```python
from build123d import *
from build123d.topology import SkipClean

# Parameters (mm, degrees)
SKETCH1_R           = 3.2512
SKETCH1_R_2         = 1.4732
SKETCH1_R_3         = 2.2987
BOSS_EXTRUDE1_DEPTH = 3.81
CUT_EXTRUDE2_START  = -1.651
CUT_EXTRUDE2_DEPTH  = 1.651


with BuildPart() as part:
    # Sketch1 → Boss-Extrude1 (new body)
    with BuildSketch(Plane.XY):
        with BuildLine():
            Line((7.944916334, 12.956699963), (-7.685191608, 2.536045689))
            ThreePointArc((-7.685191608, 2.536045689), (-9.0424, 0), (-7.685191608, -2.536045689))
            Line((-7.685191608, -2.536045689), (7.944916334, -12.956699963))
            ThreePointArc((7.944916334, -12.956699963), (13.779763951, -12.157804059), (13.70040037, -6.26905353))
            ThreePointArc((13.70040037, -6.26905353), (11.2776, 0), (13.70040037, 6.26905353))
            ThreePointArc((13.70040037, 6.26905353), (13.779763951, 12.157804059), (7.944916334, 12.956699963))
        make_face()
        with Locations(Location((0, 0, 0), (0, 0, 180))):
            Circle(SKETCH1_R, mode=Mode.SUBTRACT)
        with Locations(Location((-5.9944, 0, 0), (0, 0, 180))):
            Circle(SKETCH1_R_2, mode=Mode.SUBTRACT)
        with Locations(Location((5.9944, 0, 0), (0, 0, 180))):
            Circle(SKETCH1_R_2, mode=Mode.SUBTRACT)
        with Locations(Location((10.410654097, 9.2583, 0), (0, 0, 180))):
            Circle(SKETCH1_R_3, mode=Mode.SUBTRACT)
        with Locations(Location((10.410654097, -9.2583, 0), (0, 0, 180))):
            Circle(SKETCH1_R_3, mode=Mode.SUBTRACT)
    extrude(amount=BOSS_EXTRUDE1_DEPTH)

    # Sketch2 → Cut-Extrude2 (cut)
    with SkipClean():  # the faces are left unmerged after this step: merging them gives an invalid solid
        with BuildSketch(Plane.XY.offset(3.81).offset(CUT_EXTRUDE2_START)):
            with BuildLine():
                Line((7.944916334, 12.956699963), (-7.685191608, 2.536045689))
                ThreePointArc((-7.685191608, 2.536045689), (-9.0424, 0), (-7.685191608, -2.536045689))
                Line((-7.685191608, -2.536045689), (7.944916334, -12.956699963))
                ThreePointArc((7.944916334, -12.956699963), (7.041544243, -6.358795941), (13.70040037, -6.26905353))
                ThreePointArc((13.70040037, -6.26905353), (11.2776, 0), (13.70040037, 6.26905353))
                ThreePointArc((13.70040037, 6.26905353), (7.041544243, 6.358795941), (7.944916334, 12.956699963))
            make_face()
        extrude(amount=CUT_EXTRUDE2_DEPTH, mode=Mode.SUBTRACT)


solid = part.part
```
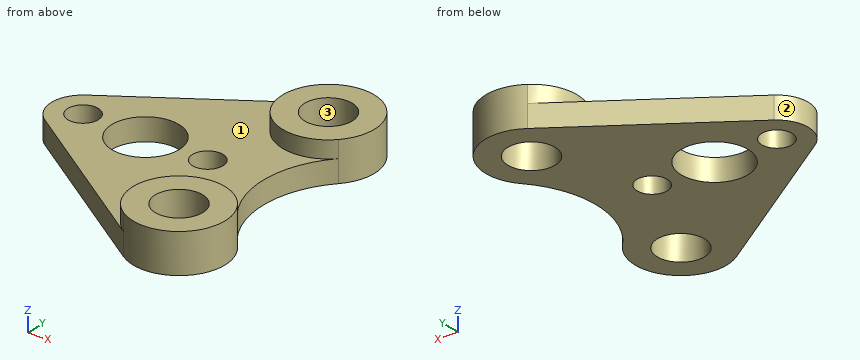
CAD build for the part. Positions are in the model's coordinates, mm. Face numbers are marked on the shaded views. Coordinates: 2 decimals unless noted, no trailing zeros. Write each loop counter-clockwise with the first axis right and the second up, starting at its lowest first coordinate (ties: lowest second). Pieces come first, ordered by that corner, then holes. Notation, with made-up numbers: (33.5, 26) -> (77.5, 26) arc R24 ccw to (77.5, 46) -> close; hole circle Ø9 at (26.5, 17.5). An arc over 180 degrees is marked (long way). Return JSON: item names as keys, results as strings. Group by question number.
Q1. Drill centre lines: line 1 (Y direction, x = 12.5, z = 2.75); line 2 (Y direction, x = 9.5, z = 2); line 3 (Y direction, x = 9.75, z = 2.5). Where is each one in solid material? Low to high.
Q2. Cut at B-B, the plane x = 10.75. Give the cut face in (y, z).
Q3. Cut at D-D, the plane x = 0. Give the cut face in (y, z).
Q4. Cut at C-C, the plane z = 3.1. Give the cut face in (x, y) (3 decimals), then the cut area to 3 significant figures.
Q5. Cut at A-A, the plane y = 0. Give the cut face in (x, z).
Q6. Flat gauge pins, fed straight in: pin 1 (1.5 mm diameter, centred on x = -3.5, z = 2.5, fed in from -Y); pin 2 (5 mm diameter, centred on x = 0, y = 0, fed in from +Z); pin 3 (1.5 mm diameter, centred on y = -1, z = 2, fed in from +X); pin 4 (7 mm diameter, centred on x = -3, y = 4.5, fed in from +Z). Where does each tip first touch, or does it go through?
Q7. Pull direction X, two halves, no side cores. Call the marked faces 1, 2 and 3: released by +X, released by -X, zero draft, split by the parting line, or undercut.
Returned:
{
 "1": {"line 1": "y = -13.18 to -10.22, -8.3 to -5.33, 5.33 to 8.3, 10.22 to 13.18", "line 2": "y = -13.61 to -11.37, -7.15 to 7.15, 11.37 to 13.61", "line 3": "y = -13.65 to -11.46, -7.06 to -4.86, 4.86 to 7.06, 11.46 to 13.65"},
 "2": {"outline": "(-13.69, 0) -> (-11.53, 0) -> (-11.53, 3.81) -> (-13.69, 3.81) -> close; (-6.98, 0) -> (6.98, 0) -> (6.98, 3.81) -> (4.83, 3.81) -> (4.83, 2.16) -> (-4.83, 2.16) -> (-4.83, 3.81) -> (-6.98, 3.81) -> close; (11.53, 0) -> (13.69, 0) -> (13.69, 3.81) -> (11.53, 3.81) -> close"},
 "3": {"outline": "(-7.66, 0) -> (-3.25, 0) -> (-3.25, 2.16) -> (-7.66, 2.16) -> close; (3.25, 0) -> (7.66, 0) -> (7.66, 2.16) -> (3.25, 2.16) -> close"},
 "4": {"outline": "circle Ø8.89 at (10.411, -9.258); circle Ø8.89 at (10.411, 9.258); hole circle Ø4.597 at (10.411, -9.258); hole circle Ø4.597 at (10.411, 9.258)", "area": "90.9 mm2"},
 "5": {"outline": "(-9.04, 0) -> (-7.47, 0) -> (-7.47, 2.16) -> (-9.04, 2.16) -> close; (-4.52, 0) -> (-3.25, 0) -> (-3.25, 2.16) -> (-4.52, 2.16) -> close; (3.25, 0) -> (4.52, 0) -> (4.52, 2.16) -> (3.25, 2.16) -> close; (7.47, 0) -> (11.28, 0) -> (11.28, 2.16) -> (7.47, 2.16) -> close"},
 "6": {"pin 1": "stops at y = -5.77", "pin 2": "passes through", "pin 3": "stops at x = 11.44", "pin 4": "stops at z = 2.16"},
 "7": {"face 1": "zero draft", "face 2": "released by -X", "face 3": "undercut"}
}
